Verification items for the finished model (mm, model axes). A direction names the side the tool comes from. Round coordinates to 2 decimals unless told otherwise and drop trailing zeros. Order: outer loops, then holes, each group sorted by start corner. A loop starts at its lowest first (then second) coordinate and runs counter-clockwise, first axis right, second up. Notation, with made-up numbers: M 35,-36.75 L 89,-36.75 A17 cw 89,-14.75 Z; hole C 67.5,48.25 d10. An arc over 180 degrees is marked long. Use one line per item in the form item = value. Start each with the question number.
Item 1: Tool access check on faces 1 (the cylindrical face through (-7.395, -27.934, 33.106)), 2 (the cylindrical face through (12.957, 4.014, -0.651)), 3 (the cylindrical face through (-29.399, -5.931, -33.106)), 4 (the flat face through (2, 2, 8)). Record the directions out of +Z, -Z, +X, -X, +Y, -Y that give a thin tool (end or side, any length) a straight path to the whole face; none if there is none.
Item 2: Release check for a two-part mould opening along X. For faces 5 (the cylindrical face through (1.166, 2.014, -1.517)), 6 (the flat face through (-5, 2, 0)), 7 (the cylindrical face through (-0.57, -15.86, -33.14)) record: +X half, -X half, draft (parallel to the pull), parting line (faces both ways), or undercut.
Item 3: Go/stop test with flat-tipped pins: pin 1 Ø7 at (y, z) = (0, -2.5) entering from -X; pin 2 Ø3 at (x, z) = (-10, 33) entering from +Y; pin 3 Ø4 at (x, y) = (13.5, 2) entering from +Z; pin 4 Ø11 at (y, z) = (-9.5, 24.5) entering from +X (3 decimals). Record where each tip stops, or that it passes through.
Item 4: Cross-section at D-D on z = 18.5. Enter the section's corners in (x, y), then the cut area to 3 significant figures.
Item 5: Thickness scan on probe 1 along X at (y, z) = (1.95, 0); probe 2 along Z at (x, y) = (-12, -3); probe 3 along X at (y, z) = (4.15, 0). Record the ranges inside material, lowest first. Write a range as [from, to].
Item 6: Cross-section at A-A on x = -22. Count the separate pieces of the cut face and the enclosed holes in it, then the cut area to 3 significant figures.
Item 7: Cross-section at C-C on x = 8. Enter the section's corners in (y, z), then the cut area to 3 significant figures.
from build123d import *

# Parameters (mm, degrees)
SKETCH1_W            = 5
SKETCH1_H            = 54
BOSS_EXTRUDE1_DEPTH  = 5
SKETCH3_W            = 16
SKETCH3_H            = 16
BOSS_EXTRUDE2_DEPTH  = 5
SKETCH6_W            = 5
SKETCH6_H            = 5
BOSS_EXTRUDE5_DEPTH  = 5
SKETCH10_W           = 30
SKETCH10_H           = 15
BOSS_EXTRUDE9_DEPTH  = 4
CUT_EXTRUDE1_DEPTH   = 2
CUT_EXTRUDE2_REACH   = 71.784
SKETCH11_R           = 5
SKETCH13_W           = 15
SKETCH13_H           = 2
BOSS_EXTRUDE10_DEPTH = 15
SKETCH4_R            = 5
CUT_EXTRUDE3_DEPTH   = 2
SKETCH14_R           = 7
CUT_EXTRUDE4_DEPTH   = 2
SKETCH16_W           = 6
SKETCH16_H           = 5
BOSS_EXTRUDE11_DEPTH = 5
BOSS_EXTRUDE12_START = -11
SKETCH17_R           = 2.5
BOSS_EXTRUDE12_DEPTH = 16
FILLET1_R            = 2


with BuildPart() as part:
    # Sketch1 → Boss-Extrude1 (new body)
    with BuildSketch(Plane(origin=(0, 0, 0), x_dir=(1, 0, 0), z_dir=(0, 1, 0))):
        with Locations((-2.5, 0)):
            Rectangle(SKETCH1_W, SKETCH1_H)
    extrude(amount=BOSS_EXTRUDE1_DEPTH)

    # Sketch3 → Boss-Extrude2 (add)
    with BuildSketch(Plane(origin=(0, 0, 0), x_dir=(1, 0, 0), z_dir=(0, 1, 0))):
        with Locations((8, 0)):
            Rectangle(SKETCH3_W, SKETCH3_H)
    extrude(amount=BOSS_EXTRUDE2_DEPTH)

    # Sketch6 → Boss-Extrude5 (add, along a direction that is not the sketch's normal)
    with BuildSketch(Plane.XY.offset(27)):
        with Locations((-2.5, 2.5)):
            Rectangle(SKETCH6_W, SKETCH6_H)
    boss_extrude5 = extrude(amount=BOSS_EXTRUDE5_DEPTH, dir=(0, -0.7071067811865479, 0.7071067811865472))

    # Sketch10 → Boss-Extrude9 (add)
    with BuildSketch(Plane.XY.offset(30.535533906)):
        with Locations((-15, -6.035533906)):
            Rectangle(SKETCH10_W, SKETCH10_H)
    boss_extrude9 = extrude(amount=BOSS_EXTRUDE9_DEPTH)

    # Sketch12 → Cut-Extrude1 (cut)
    with BuildSketch(Plane(origin=(0, 0, 30.535533906), x_dir=(-1, 0, 0), z_dir=(0, 0, -1))):
        Polygon((30, -13.535533906), (30, 1.464466094), (5, 1.464466094), (5, -3.535533906), (0, -3.535533906), (0, -13.535533906), align=None)
    cut_extrude1 = extrude(amount=-CUT_EXTRUDE1_DEPTH, mode=Mode.SUBTRACT)

    # Sketch11 → Cut-Extrude2 (cut, up to next)
    with BuildSketch(Plane.XY.offset(34.535533906), mode=Mode.PRIVATE) as cut_extrude2_sk1:
        with Locations((-22, -6.035533906)):
            Circle(SKETCH11_R)
    cut_extrude2_tool1 = extrude(cut_extrude2_sk1.sketch, amount=-CUT_EXTRUDE2_REACH, mode=Mode.PRIVATE) & part.part
    cut_extrude2 = cut_extrude2_tool1.solids().sort_by_distance((-22, -6.035534, 34.535534))[0]
    add(cut_extrude2, mode=Mode.SUBTRACT)

    # Sketch13 → Boss-Extrude10 (add)
    with BuildSketch(Plane.XZ.offset(13.535533906)):
        with Locations((-7.5, 33.535533906)):
            Rectangle(SKETCH13_W, SKETCH13_H)
    boss_extrude10 = extrude(amount=BOSS_EXTRUDE10_DEPTH)

    # Sketch4 → Cut-Extrude3 (cut)
    with BuildSketch(Plane(origin=(0, 5, 0), x_dir=(1, 0, 0), z_dir=(0, 1, 0))):
        with Locations(Location((8, 0, 0), (0, 0, 270))):
            Circle(SKETCH4_R)
    extrude(amount=-CUT_EXTRUDE3_DEPTH, mode=Mode.SUBTRACT)

    # Sketch14 → Cut-Extrude4 (cut)
    with BuildSketch(Plane(origin=(0, 3, 0), x_dir=(1, 0, 0), z_dir=(0, 1, 0))):
        with Locations(Location((8, 0, 0), (0, 0, 270))):
            Circle(SKETCH14_R)
    extrude(amount=-CUT_EXTRUDE4_DEPTH, mode=Mode.SUBTRACT)

    # Sketch16 → Boss-Extrude11 (add)
    with BuildSketch(Plane.XY.offset(8)):
        with Locations((8, 2.5)):
            Rectangle(SKETCH16_W, SKETCH16_H)
    boss_extrude11 = extrude(amount=BOSS_EXTRUDE11_DEPTH)

    # Sketch17 → Boss-Extrude12 (add)
    with BuildSketch(Plane(origin=(11, 0, 0), x_dir=(0, 0, -1), z_dir=(1, 0, 0)).offset(BOSS_EXTRUDE12_START)):
        with Locations((-13, 2.5)):
            Circle(SKETCH17_R)
    boss_extrude12 = extrude(amount=BOSS_EXTRUDE12_DEPTH)

    # Mirror2: Boss-Extrude5, Boss-Extrude9, Cut-Extrude1, Cut-Extrude2, Boss-Extrude10, Boss-Extrude11, Boss-Extrude12 across plane
    add(boss_extrude5.mirror(Plane.XY))
    add(boss_extrude9.mirror(Plane.XY))
    add(cut_extrude1.mirror(Plane.XY), mode=Mode.SUBTRACT)
    add(cut_extrude2.mirror(Plane.XY), mode=Mode.SUBTRACT)
    add(boss_extrude10.mirror(Plane.XY))
    add(boss_extrude11.mirror(Plane.XY))
    add(boss_extrude12.mirror(Plane.XY))

    # Fillet1
    fillet1_edges = [part.edges().sort_by_distance(p)[0] for p in [
        (0, -16.035533906, -32.535533906),
        (0, -16.035533906, 32.535533906),
        (-7.5, -28.535533906, 32.535533906),
        (-17.5, 1.464466094, -32.535533906),
        (-30, -6.035533906, -32.535533906),
        (-22.5, -13.535533906, -32.535533906),
        (-15, -21.035533906, -32.535533906),
        (-7.5, -28.535533906, -32.535533906),
        (-17.5, 1.464466094, 32.535533906),
        (-30, -6.035533906, 32.535533906),
        (-22.5, -13.535533906, 32.535533906),
        (-15, -21.035533906, 32.535533906),
    ]]
    fillet(fillet1_edges, radius=FILLET1_R - 0.0001)  # a hair under: the kernel refuses the full size


solid = part.part
Output values:
q1.face_1 = +X, -X, -Y
q1.face_2 = +Y
q1.face_3 = -X, +Y, -Y
q1.face_4 = +Y, -Y
q2.face_5 = undercut
q2.face_6 = -X half
q2.face_7 = +X half
q3.pin_1 = -5
q3.pin_2 = 1.46
q3.pin_3 = 15.5
q3.pin_4 = through
q4.outline = M -5,0 L 0,0 L 0,5 L -5,5 Z
q4.area = 25.0 mm2
q5.probe_1 = [-5, 1], [15, 16]
q5.probe_2 = [-34.54, -32.54], [32.54, 34.54]
q5.probe_3 = [-5, 3], [13, 16]
q6.separate_pieces = 4
q6.enclosed_holes = 0
q6.area = 16.6 mm2
q7.outline = M 0,-13 A2.5 ccw 5,-13 L 5,-5 L 3,-5 L 3,-7 L 1,-7 L 1,7 L 3,7 L 3,5 L 5,5 L 5,13 A2.5 ccw 0,13 Z
q7.area = 102 mm2
